```python
from build123d import *

# Parameters (mm, degrees)
SKETCH1_W           = 94.294111711
SKETCH1_H           = 123.247490411
BOSS_EXTRUDE1_DEPTH = 41
SKETCH2_W           = 123.247490411
SKETCH2_H           = 11.729493647
BOSS_EXTRUDE2_DEPTH = 115
SKETCH3_W           = 115
SKETCH3_H           = 11.729493647
BOSS_EXTRUDE3_DEPTH = 115


with BuildPart() as part:
    # Sketch1 → Boss-Extrude1 (new body)
    with BuildSketch(Plane(origin=(0, 0, 0), x_dir=(1, 0, 0), z_dir=(0, 1, 0))):
        with Locations((47.147055855, 61.623745206)):
            Rectangle(SKETCH1_W, SKETCH1_H)
    extrude(amount=BOSS_EXTRUDE1_DEPTH)

    # Sketch2 → Boss-Extrude2 (add)
    with BuildSketch(Plane.ZY):
        with Locations((-61.623745206, 5.864746823)):
            Rectangle(SKETCH2_W, SKETCH2_H)
    extrude(amount=BOSS_EXTRUDE2_DEPTH)

    # Sketch3 → Boss-Extrude3 (add)
    with BuildSketch(Plane(origin=(0, 0, -123.247490411), x_dir=(-1, 0, 0), z_dir=(0, 0, -1))):
        Polygon((-94.294111711, 41), (-94.294111711, 0), (0, 0), (0, 11.729493647), (0, 41), align=None)
        with Locations((57.5, 5.864746823)):
            Rectangle(SKETCH3_W, SKETCH3_H)
    extrude(amount=BOSS_EXTRUDE3_DEPTH)


solid = part.part
```
Work out the finished part from the listing and answer in its coordinate system (mm). A direction names the side the tool comes from. Round coordinates to 2 decimals unless told otherwise and drop trailing zeros. Write each loop counter-clockwise with the first axis right and the second up, starting at its lowest first coordinate (ties: lowest second). Pieces come first, ordered by that corner, then holes.
1) Consider probe 1 along X at (y, z) = (32, -227); probe 2 along Y at (x, z) = (-94, -205). Determine where each line is inside the solid, lowest interval first.
2) A cutting plane is placed at A-A on z = -151. Determine the outline of the cut face in (x, y), and give its area (3 significant figures).
3) Which of the six approach directions +Z, -Z, +X, -X, +Y, -Y give full straight-line access (tool end or side, diameter ignored) to faces 1 (the face through (14, 16, -238.247)), 2 (the face through (-57, 11.729, -117))?
4) A cutting plane is placed at C-C on x = -57.5. Determine the outline of the cut face in (y, z).
5) A cutting plane is placed at B-B on y = 38. Determine the outline of the cut face in (x, z).
6) A flat-ended cylindrical pin translates along its axis: P1, Ø14.5, axis at y = 33.5, z = -109, coming from the -X side. Find the tip coordinate at first contact, or state that the pin passes through.
Entries:
1. probe 1: x = 0 to 94.29
1. probe 2: y = 0 to 11.73
2. outline: (-115, 0) - (94.29, 0) - (94.29, 41) - (0, 41) - (0, 11.73) - (-115, 11.73) - close
2. area: 5,210 mm2
3. face 1: -Z, +X, -X, +Y, -Y
3. face 2: +Z, -Z, -X, +Y
4. outline: (0, -238.25) - (11.73, -238.25) - (11.73, 0) - (0, 0) - close
5. outline: (0, -238.25) - (94.29, -238.25) - (94.29, 0) - (0, 0) - close
6. P1: stops at x = 0
